Work out the finished part from the listing and answer in its coordinate system (mm). Face numbers are marked on the shaded views. A direction names the side the tool comes from. Coordinates: 2 decimals unless noted, no trailing zeros. Loops run counter-clockwise (first coordinate to the right, second up) from the corner with the lowest first, then second, coordinate; pieces in that order, holes last. Notation, with made-up numbers: (62, 6.5) -> (108, 6.5) arc R21 cw to (108, 13.5) -> close; hole circle Ø8 at (3.5, 31.5). An arc over 180 degrees is marked (long way). One line per question, with ' | ' between items.
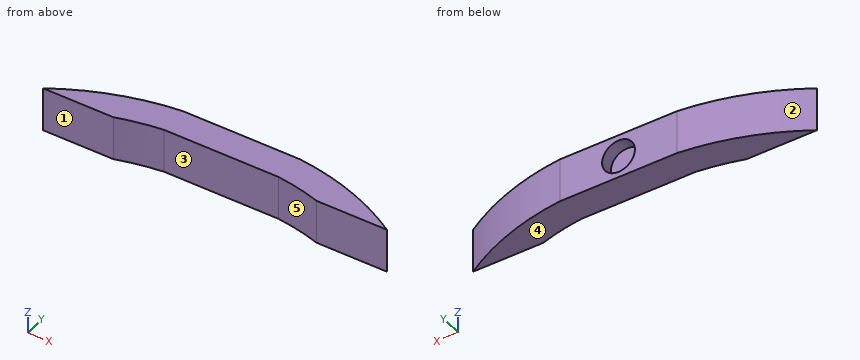
```python
from build123d import *

# Parameters (mm, degrees)
BOSS_EXTRUDE1_DEPTH = 10.16
SKETCH2_R           = 3.81
CUT_EXTRUDE1_DEPTH  = 3


with BuildPart() as part:
    # Sketch1 → Boss-Extrude1 (new body)
    with BuildSketch(Plane.XY):
        with BuildLine():
            Line((-13.62, 60.264846167), (13.62, 60.264846167))
            ThreePointArc((13.62, 60.264846167), (27.323058228, 57.250841389), (39.965, 51.164846167))
            Line((39.965, 51.164846167), (23.620484036, 51.164846167))
            ThreePointArc((23.620484036, 51.164846167), (18.493954537, 52.501006754), (13.260607764, 53.324846167))
            Line((13.260607764, 53.324846167), (-13.260607764, 53.324846167))
            ThreePointArc((-13.260607764, 53.324846167), (-18.493954537, 52.501006754), (-23.620484036, 51.164846167))
            Line((-23.620484036, 51.164846167), (-39.965, 51.164846167))
            ThreePointArc((-39.965, 51.164846167), (-27.323058228, 57.250841389), (-13.62, 60.264846167))
        make_face()
    extrude(amount=BOSS_EXTRUDE1_DEPTH)

    # Sketch2 → Cut-Extrude1 (cut)
    with BuildSketch(Plane(origin=(0, 60.264846167, 0), x_dir=(1, 0, 0), z_dir=(0, 1, 0))):
        with Locations((0, -5.08)):
            Circle(SKETCH2_R)
    extrude(amount=-CUT_EXTRUDE1_DEPTH, mode=Mode.SUBTRACT)


solid = part.part
```
1) Find section C-C (y = 54.5). Write down the section's boundary in (x, z).
Check values:
outline: (-33.98, 0) -> (33.98, 0) -> (33.98, 10.16) -> (-33.98, 10.16) -> close
2) Find section A-A (z = 5.08). Write down the section's boundary in (x, y) (3 decimals), plus the area to 3 significant figures.
Check values:
outline: (-39.965, 51.165) -> (-23.62, 51.165) arc R53.63 cw to (-13.261, 53.325) -> (13.261, 53.325) arc R53.63 cw to (23.62, 51.165) -> (39.965, 51.165) arc R60.57 ccw to (13.62, 60.265) -> (3.81, 60.265) -> (3.81, 57.265) -> (-3.81, 57.265) -> (-3.81, 60.265) -> (-13.62, 60.265) arc R60.57 ccw to start | area: 442 mm^2
3) Find the intervals of material crossed by line 1 along Z through (x, y) = (0, 58.25); line 2 along Y through (x, z) = (2.5, 7.75); line 3 along Y through (x, z) = (-3.5, 2.75), in increasing order.
Check values:
line 1: z = 0 to 1.27, 8.89 to 10.16 | line 2: y = 53.32 to 57.26 | line 3: y = 53.32 to 60.26
4) Flat-ended cylindrical pins translate along their axes: pin 1 (4 mm diameter, centred on y = 54.5, z = 6, fed in from +X); pin 2 (2 mm diameter, centred on x = 11, z = 8, fed in from -Y). Find the tip coordinate at first contact, or state that the pin passes through.
Check values:
pin 1: stops at x = 37.75 | pin 2: stops at y = 53.32
5) Find section D-D (x = 30.5). Write down the section's boundary in (y, z).
Check values:
outline: (51.16, 0) -> (56.05, 0) -> (56.05, 10.16) -> (51.16, 10.16) -> close
6) For the marked faces 4 and 5, determine the directions among +Z, -Z, +X, -X, +Y, -Y from which every point of the face is accessible in a straight line to the end or side of a thin tool.
Check values:
face 4: -Z, +X, -X, +Y, -Y | face 5: +Z, -Z, -Y
7) Find section B-B (x = 0). Write down the section's boundary in (y, z).
Check values:
outline: (53.32, 0) -> (60.26, 0) -> (60.26, 1.27) -> (57.26, 1.27) -> (57.26, 8.89) -> (60.26, 8.89) -> (60.26, 10.16) -> (53.32, 10.16) -> close
8) The mould has two halves that part along X. Classify the marked faces 1, 2 and 3: released by +X, released by -X, zero draft, split by the parting line, or undercut.
Check values:
face 1: zero draft | face 2: released by -X | face 3: undercut
